Design review of the part built by this model. Coordinates are the model's own, in mm. A direction names the side the tool comes from. Give positions to 0.01 mm unless a question says otherwise; leave off trailing zeros. Write each loop counter-clockwise with the first axis right and the second up, starting at its lowest first coordinate (ties: lowest second). Pieces come first, ordered by that corner, then holes. Notation, with made-up numbers: (-35.5, -10.75) -> (-12.5, -10.75) arc R19 cw to (-12.5, 6.25) -> close; hole circle Ø1 at (21, -38.5). An arc over 180 degrees is marked (long way). Return JSON: item names as keys, results as strings. Group by question number.
from build123d import *

# Parameters (mm, degrees)
F0_W     = 54
F0_H     = 94
F1_DEPTH = 710
F3_START = 20
F3_DEPTH = 35
F4_START = 20
F4_DEPTH = 35


with BuildPart() as f1:
    # F0 (on Right) → F1 (new body, symmetric)
    with BuildSketch(Plane.YZ):
        with BuildLine():
            ThreePointArc((30, 47), (29.1213203436, 49.1213203436), (27, 50))
            Line((27, 50), (-27, 50))
            ThreePointArc((-27, 50), (-29.1213203436, 49.1213203436), (-30, 47))
            Line((-30, 47), (-30, -47))
            ThreePointArc((-30, -47), (-29.1213203436, -49.1213203436), (-27, -50))
            Line((-27, -50), (27, -50))
            ThreePointArc((27, -50), (29.1213203436, -49.1213203436), (30, -47))
            Line((30, -47), (30, 47))
        make_face()
        Rectangle(F0_W, F0_H, mode=Mode.SUBTRACT)
    extrude(amount=F1_DEPTH, both=True)

    # F2 (on Top) → F3 (cut)
    with BuildSketch(Plane.XY.offset(F3_START)):
        with BuildLine():
            Line((-590.61, 40), (-662.61, 40))
            Line((-662.61, 40), (-662.61, 14))
            ThreePointArc((-662.61, 14), (-665.4384271247, 7.1715728753), (-658.61, 10))
            Line((-658.61, 10), (-594.61, 10))
            ThreePointArc((-594.61, 10), (-587.7815728753, 7.1715728753), (-590.61, 14))
            Line((-590.61, 14), (-590.61, 40))
        make_face()
    extrude(amount=F3_DEPTH, mode=Mode.SUBTRACT)

    # F2 (on Top) → F4 (cut)
    with BuildSketch(Plane.XY.offset(F4_START)):
        with BuildLine():
            Line((662.61, 14), (662.61, 40))
            Line((662.61, 40), (590.61, 40))
            Line((590.61, 40), (590.61, 14))
            ThreePointArc((590.61, 14), (587.7815728753, 7.1715728753), (594.61, 10))
            Line((594.61, 10), (658.61, 10))
            ThreePointArc((658.61, 10), (665.4384271247, 7.1715728753), (662.61, 14))
        make_face()
    extrude(amount=F4_DEPTH, mode=Mode.SUBTRACT)


solid = f1.part
Q1. Take a section at D-D, the plane x = -607.5. Give the boundary of the cut face in (y, z), plus the area to 3 significant figures.
Q2. For L1, parallel to Y at x = -493, z = 3; L2, parallel to Z at x = -226, y = -14; L3, parallel to Y at x = -590, z = 49, list the stretches that pass through material, from the lowest coordinate up. Write a range as from..to.
Q3. Mouldability with a two-part tool opening along Z and no side actions: class faces 1 (the face through (10, 0, 50)), 2 (the face through (-710, -29, 0)), 3 (the face through (10, 27, -1)) as +Z half, -Z half, draft (parallel to the pull), parting line (faces both ways), or undercut.
Q4. Take a section at A-A, the plane z = -3.5. Give the boundary of the cut face in (x, y).
Q5. Tool access review of faces 4 (the face through (10, 30, -1)), 5 (the face through (10, 0, -47)): name each direction out of +Z, -Z, +X, -X, +Y, -Y from which nothing blocks a thin tool from reaching the whole face with its end or side.
Q6. Insertion check: pin 1 (3.5 mm diameter, centred on x = -622, z = 48.5, fed in from +Y); pin 2 (0.9 mm diameter, centred on x = -608.5, y = 28, fed in from +Z). Each pin has a flat end and moves straight along its axis. Give the tip position at first contact, or say it passes through.
Q7. Take a section at B-B, the plane x = 117. Give the boundary of the cut face in (y, z), plus the area to 3 significant figures.
Q8. Take a section at C-C, the plane y = -15. Give the boundary of the cut face in (x, z).
Final values:
{
 "1": {"outline": "(-30, -47) arc R3 ccw to (-27, -50) -> (27, -50) arc R3 ccw to (30, -47) -> (30, 20) -> (27, 20) -> (27, -47) -> (-27, -47) -> (-27, 47) -> (10, 47) -> (10, 50) -> (-27, 50) arc R3 ccw to (-30, 47) -> close", "area": "777 mm²"},
 "2": {"L1": "y = -30..-27, 27..30", "L2": "z = -50..-47, 47..50", "L3": "y = -29.24..6.05, 13.95..29.24"},
 "3": {"face 1": "+Z half", "face 2": "draft", "face 3": "undercut"},
 "4": {"outline": "(-710, -30) -> (710, -30) -> (710, -27) -> (-710, -27) -> close; (-710, 27) -> (710, 27) -> (710, 30) -> (-710, 30) -> close"},
 "5": {"face 4": "+Z, -Z, +X, -X, +Y", "face 5": "+X, -X"},
 "6": {"pin 1": "stops at y = 10", "pin 2": "stops at z = 20"},
 "7": {"outline": "(-30, -47) arc R3 ccw to (-27, -50) -> (27, -50) arc R3 ccw to (30, -47) -> (30, 47) arc R3 ccw to (27, 50) -> (-27, 50) arc R3 ccw to (-30, 47) -> close; hole (-27, -47) -> (27, -47) -> (27, 47) -> (-27, 47) -> close", "area": "916 mm²"},
 "8": {"outline": "(-710, -50) -> (710, -50) -> (710, -47) -> (-710, -47) -> close; (-710, 47) -> (710, 47) -> (710, 50) -> (-710, 50) -> close"}
}
